For this review, take the finished solid that the model builds, in its own axes (mm). A direction names the side the tool comes from. Round coordinates to 2 decimals unless told otherwise and drop trailing zeros. Write each loop counter-clockwise with the first axis right and the second up, starting at its lowest first coordinate (ties: lowest second). Pieces come first, ordered by that corner, then holes. Notation, with made-up numbers: (53, 7.5) -> (110, 7.5) arc R11 ccw to (110, 12.5) -> close; hole circle Ø10 at (-2, 57.25). An arc over 180 degrees is marked (long way). Answer in a Markdown table with one row per item.
Solid Edge part; units mm, degrees
sketch "Sketch1" plane through (0, 0, 0) normal (0, -1, 0) x (1, 0, 0)
  line L0 (0, 0) -> (0, 220)
  arc A0 (0, 220) -> (80, 300) centre (80, 220) cw
  line L1 (80, 300) -> (270, 300)
  arc A1 (270, 300) -> (350, 220) centre (270, 220) cw
  line L2 (350, 220) -> (350, 0)
sketch "Sketch2" plane through (0, 0, 0) normal (0, 0, -1) x (-1, 0, 0)
  circle A0 centre (0, 0) radius 9.5
sweep "SweptProtrusion_1" add profiles "Sketch2" path "Sketch1"
shell "Thinwall_1" thickness 1.6 removed faces 4 at (6.5233, -6.1433, 0) at (343.4767, -6.1433, 0) at (6.5233, -6.1433, 0) at (343.4767, -6.1433, 0)
hole "Hole_1" at (0, 0, 0) direction (0, -1, 0) diameter 19 end through all both ways yes
hole "Hole1" at (350, 0, 0) direction (0, -1, 0) diameter 19 end through all both ways yes
properties material "Aluminum, 1060"
1) Mouldability with a two-part tool opening along Y and no side actions: class faces 4 (the cylindrical face through (7, -6.42, 111.54)), 5 (the cylindrical face through (357.535, -2.373, 111.134)) as pulls with the +Y half, pulls with the -Y half, needs draft (parallel to the pull), parting line crosses it, or undercut.
Solved:
| item | result |
|---|---|
| face 4 | parting line crosses it |
| face 5 | undercut |
2) Consider section B-B on z = 164. State the section outline as (x, y) points, then the cut area to 3 significant figures.
Solved:
| item | result |
|---|---|
| outline | circle Ø19 at (0, 0); circle Ø19 at (350, 0); hole circle Ø15.8 at (0, 0); hole circle Ø15.8 at (350, 0) |
| area | 175 mm² |
3) Consider section C-C on x = 124. State the section outline as (y, z) points, then the cut area to 3 significant figures.
Solved:
| item | result |
|---|---|
| outline | circle Ø19 at (0, 300); hole circle Ø15.8 at (0, 300) |
| area | 87.5 mm² |
4) For faces 1 (the cylindrical face through (176.33, -2.373, 307.535)), 2 (the cylindrical face through (6.269, 4.807, 114.14)), 3 (the cylindrical face through (-7.6, 2.8, 5.7)), list the 3-axis set-ups (+Z, -Z, +X, -X, +Y, -Y) from which the entire face can be reached by the end or side of a thin tool; tool diameter is ignored.
Solved:
| item | result |
|---|---|
| face 1 | none |
| face 2 | -Z |
| face 3 | -Z, +Y, -Y |
5) For line 1 (X direction, y = 0, z = 110); line 2 (Y direction, x = 161, z = 300); line 3 (Z direction, x = 133, y = 0), list the stretches that pass through material, from the lowest coordinate up. Write a range as [from, to].
Solved:
| item | result |
|---|---|
| line 1 | [-9.5, -7.9], [7.9, 9.5], [340.5, 342.1], [357.9, 359.5] |
| line 2 | [-9.5, -7.9], [7.9, 9.5] |
| line 3 | [290.5, 292.1], [307.9, 309.5] |
6) Clearance check with flat-ended pins moving along their axes: pin 1 Ø10 at (x, y) = (281.5, 3.5) entering from +Z; pin 2 Ø10 at (y, z) = (-5.5, 263) entering from +X; pin 3 Ø9.5 at (y, z) = (0, 300) entering from -X. State where each tip first meets the part, or that it passes through.
Solved:
| item | result |
|---|---|
| pin 1 | z = 309.17 |
| pin 2 | x = 350.19 |
| pin 3 | x = 31.55 |
